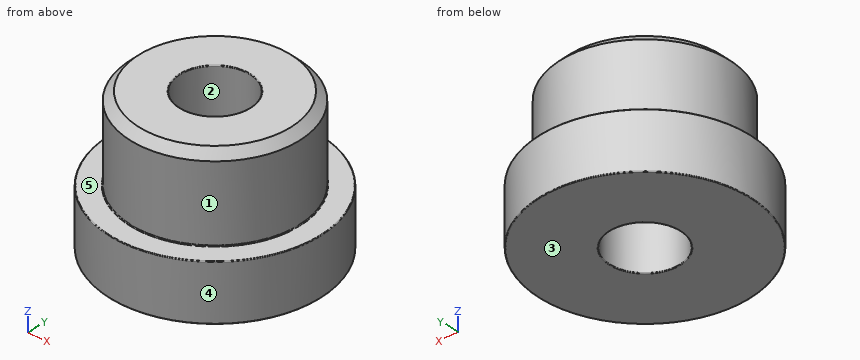
from build123d import *

# Parameters (mm, degrees)
F2_R    = 0.25
F3_SIZE = 3


with BuildPart() as f1:
    # F0 (on Front) → F1 (revolve)
    with BuildSketch(Plane.XZ):
        Polygon((30, 50), (12.5, 50), (12.5, 0), (37.5, 0), (37.5, 20), (30, 20), align=None)
    revolve(axis=Axis((0, 0, 16.379672), (0, 0, -1)))

    # F2
    f2_edges = [f1.edges().sort_by_distance(p)[0] for p in [
        (-12.5, 0, 50),
        (-12.5, 0, 0),
        (12.5, 0, 25),
        (-37.5, 0, 20),
        (-30, 0, 20),
        (-37.5, 0, 0),
    ]]
    fillet(f2_edges, radius=F2_R)

    # F3
    f3_edges = [f1.edges().sort_by_distance(p)[0] for p in [
        (-30, 0, 50),
    ]]
    chamfer(f3_edges, length=F3_SIZE)


solid = f1.part
Source: CAD feature listing. Evaluate the final solid. Frame: model axes, mm. Face numbers are marked on the shaded views. A direction names the side the tool comes from. Coordinates: 2 decimals unless noted, no trailing zeros. Order: outer loops, then holes, each group sorted by start corner. A loop starts at its lowest first (then second) coordinate and runs counter-clockwise, first axis right, second up. Notation, with made-up numbers: M -27,32.5 L 9,32.5 A18 cw 9,43.5 Z; hole C 70,31.5 d6. An arc over 180 degrees is marked long. Write each question's results on one line, items separated by ' | '. Start each with the question number.
Item 1: Cut plane D-D (z = 33). Return loops of the section in (x, y), and give its area (3 significant figures).
Item 2: First-contact query: pin 1 Ø6 at (x, z) = (-19, 37) entering from -Y; pin 2 Ø6 at (x, z) = (-14.5, 31) entering from +Y; pin 3 Ø1 at (y, z) = (0.5, 37.5) entering from +X. Flat tips, straight axial feed; report the tip coordinate or a pass-through.
Item 3: Draft query along X for the marked faces 1, 2 and 3. Return one class per face: pulls with the +X half, pulls with the -X half, needs draft (parallel to the pull), parting line crosses it, or undercut.
Item 4: Cut plane C-C (z = 5). Return loops of the section in (x, y), and give its area (3 significant figures).
Item 5: Cut plane A-A (y = 0). Return loops of the section in (x, z).
Item 6: Line query: probe 1 along Y at (x, z) = (0, 28); probe 2 along Z at (x, y) = (29, -20); probe 3 along Y at (x, z) = (0, 19). Output: solid intervals per line, ascending.
Item 7: Set-up query: the marked faces 4 and 5. Return all of +Z, -Z, +X, -X, +Y, -Y with unobstructed straight access to the full face (end or side cutting, diameter ignored); none if empty.
Checked values:
1) outline: C 0,0 d60; hole C 0,0 d25 | area: 2,340 mm2
2) pin 1: stops at y = -25.38 | pin 2: stops at y = 27.71 | pin 3: stops at x = 30
3) face 1: parting line crosses it | face 2: undercut | face 3: needs draft
4) outline: C 0,0 d75; hole C 0,0 d25 | area: 3,930 mm2
5) outline: M -37.5,0.25 A0.25 ccw -37.25,0 L -12.75,0 A0.25 ccw -12.5,0.25 L -12.5,49.75 A0.25 ccw -12.75,50 L -27,50 L -30,47 L -30,20.25 A0.25 cw -30.25,20 L -37.25,20 A0.25 ccw -37.5,19.75 Z; M 12.5,0.25 A0.25 ccw 12.75,0 L 37.25,0 A0.25 ccw 37.5,0.25 L 37.5,19.75 A0.25 ccw 37.25,20 L 30.25,20 A0.25 cw 30,20.25 L 30,47 L 27,50 L 12.75,50 A0.25 ccw 12.5,49.75 Z
6) probe 1: y = -30 to -12.5, 12.5 to 30 | probe 2: z = 0 to 20 | probe 3: y = -37.5 to -12.5, 12.5 to 37.5
7) face 4: +Z, -Z | face 5: +Z
